For this review, take the finished solid that the model builds, in its own axes (mm). A direction names the side the tool comes from. Round coordinates to 2 decimals unless told otherwise and drop trailing zeros. Order: outer loops, then holes, each group sorted by start corner. A loop starts at its lowest first (then second) coordinate and runs counter-clockwise, first axis right, second up.
from build123d import *

# Parameters (mm, degrees)
F0_W     = 101.6
F0_H     = 101.6
F1_DEPTH = 101.6
F3_DEPTH = 76.2
F4_W     = 50.8
F4_H     = 12.7
F5_DEPTH = 76.2
F6_W     = 12.7
F6_H     = 25.4
F7_DEPTH = 68.326


with BuildPart() as f1:
    # F0 (on Right) → F1 (new body)
    with BuildSketch(Plane.YZ):
        with Locations((50.8, -50.8)):
            Rectangle(F0_W, F0_H)
    extrude(amount=-F1_DEPTH)

    # F2 (on face) → F3 (cut)
    with BuildSketch(Plane.XY):
        Polygon((-76.2, 63.5), (-101.6, 63.5), (-101.6, 0), (0, 0), (0, 63.5), (-25.4, 63.5), align=None)
    extrude(amount=-F3_DEPTH, mode=Mode.SUBTRACT)

    # F4 (on face) → F5 (cut)
    with BuildSketch(Plane.XY):
        with Locations((-50.8, 69.85)):
            Rectangle(F4_W, F4_H)
    extrude(amount=-F5_DEPTH, mode=Mode.SUBTRACT)

    # F6 (on face) → F7 (cut)
    with BuildSketch(Plane.XY.offset(-76.2)):
        Polygon((-101.6, 25.4), (-101.6, 0), (-76.2, 0), align=None)
        Polygon((0, 0), (0, 25.4), (-25.4, 0), align=None)
        with Locations((-57.15, 38.1)):
            Rectangle(F6_W, F6_H)
        with Locations((-44.45, 38.1)):
            Rectangle(F6_W, F6_H)
    extrude(amount=-F7_DEPTH, mode=Mode.SUBTRACT)


solid = f1.part
(1) Draft analysis for pull direction Y (two halves, no side actions). For faces 1 (the face through (-50, 101.6, -52)), 2 (the face through (-50, 61, -101.6)), 3 (the face through (-63.5, 38, -89)), state which applies: pulls with the +Y half, pulls with the -Y half, needs draft (parallel to the pull), parting line crosses it, or undercut.
(2) Wall thickness on L1, parallel to X at y = 71, z = -72; L2, parallel to Z at x = -21, y = 48; L3, parallel to Y at x = -36.5, z = -24: over which ranges is each line inside the solid? List them lowest first.
(3) Clearance check with flat-ended pins moving along their axes: P1, Ø4, axis at x = -38, z = -69.5, coming from the -Y side; P2, Ø20.5, axis at x = -88, z = -53, coming from the -Y side. State where each tip first meets the part, or that it passes through.
(4) Add section D-D on z = -7. Give the boundary of the cut face in (x, y), plus the area to 3 significant figures.
(5) Add section B-B on x = -42.5. Give the boundary of the cut face in (y, z), plus the area to 3 significant figures.
(6) Add section C-C on z = -82. Give the boundary of the cut face in (x, y), plus the area to 3 significant figures.
(7) Tool access review of faces 4 (the face through (-51, 50.8, -89)), 5 (the face through (0, 80, -61)), 6 (the face through (-89, 63.5, -38)), 7 (the face through (-25.4, 70, -38)): name each direction out of +Z, -Z, +X, -X, +Y, -Y from which nothing blocks a thin tool from reaching the whole face with its end or side.
(8) Add section A-A on y = 49. Give the boundary of the cut face in (x, z).
Here are the results:
1. face 1: pulls with the +Y half
1. face 2: needs draft
1. face 3: undercut
2. L1: x = -101.6 to -76.2, -25.4 to 0
2. L2: z = -101.6 to -76.2
2. L3: y = 76.2 to 101.6
3. P1: stops at y = 76.2
3. P2: stops at y = 63.5
4. outline: (-101.6, 63.5) - (-76.2, 63.5) - (-76.2, 76.2) - (-25.4, 76.2) - (-25.4, 63.5) - (0, 63.5) - (0, 101.6) - (-101.6, 101.6) - close
4. area: 3,230 mm2
5. outline: (0, -101.6) - (25.4, -101.6) - (25.4, -76.2) - (0, -76.2) - close; (50.8, -101.6) - (101.6, -101.6) - (101.6, 0) - (76.2, 0) - (76.2, -76.2) - (50.8, -76.2) - close
5. area: 3,870 mm2
6. outline: (-101.6, 25.4) - (-76.2, 0) - (-25.4, 0) - (0, 25.4) - (0, 101.6) - (-101.6, 101.6) - close; hole (-63.5, 25.4) - (-38.1, 25.4) - (-38.1, 50.8) - (-63.5, 50.8) - close
6. area: 9,030 mm2
7. face 4: +Z, -Z
7. face 5: +Z, -Z, +X, +Y, -Y
7. face 6: +Z, +X, -X, -Y
7. face 7: +Z, -Y
8. outline: (-101.6, -101.6) - (-63.5, -101.6) - (-63.5, -76.2) - (-101.6, -76.2) - close; (-38.1, -101.6) - (0, -101.6) - (0, -76.2) - (-38.1, -76.2) - close
